from build123d import *

# Parameters (mm, degrees)
SKETCH1_W                 = 40
SKETCH1_H                 = 20
BOSS_EXTRUDE1_DEPTH       = 38
BOSS_EXTRUDE2_DEPTH       = 2
BOSS_EXTRUDE3_DEPTH       = 0.5
SKETCH6_W                 = 12.8
SKETCH6_H                 = 17.8
SKETCH6_W_2               = 10.8
SKETCH6_H_2               = 15.8
BOSS_EXTRUDE4_DEPTH       = 0.5
BOSS_EXTRUDE5_DEPTH       = 0.5
SKETCH8_R                 = 6.5
BOSS_EXTRUDE6_DEPTH       = 1
SKETCH9_R                 = 5.25
BOSS_EXTRUDE7_DEPTH       = 0.5
SKETCH10_R                = 3
BOSS_EXTRUDE8_DEPTH       = 4
SKETCH11_R                = 1.5
CUT_EXTRUDE1_DEPTH        = 10
CHAMFER1_SIZE             = 2
SKETCH12_R                = 2
CUT_EXTRUDE2_DEPTH        = 2
FILLET1_R                 = 0.5
FILLET2_R                 = 0.25
BOSS_EXTRUDE9_DEPTH       = 2.4
BOSS_EXTRUDE10_DEPTH      = 0.5
BOSS_EXTRUDE10_DEPTH_BACK = 0.5
FILLET3_R                 = 1.5


with BuildPart() as part:
    # Sketch1 → Boss-Extrude1 (new body)
    with BuildSketch(Plane(origin=(0, 0, 0), x_dir=(1, 0, 0), z_dir=(0, 1, 0))):
        Rectangle(SKETCH1_W, SKETCH1_H)
    extrude(amount=BOSS_EXTRUDE1_DEPTH)

    # Sketch2 → Boss-Extrude2 (add)
    with BuildSketch(Plane(origin=(0, 38, 0), x_dir=(1, 0, 0), z_dir=(0, 1, 0))):
        with BuildLine():
            ThreePointArc((-3.783333333, 0), (-7.418581742, 5.77726026), (-14.2, 5))
            Line((-14.2, 5), (-14.2, -5))
            ThreePointArc((-14.2, -5), (-7.418581742, -5.77726026), (-3.783333333, 0))
        make_face()
        with BuildLine():
            Line((-14.2, -5), (-14.2, 5))
            ThreePointArc((-14.2, 5), (-16.6, 0), (-14.2, -5))
        make_face()
        with BuildLine():
            Line((5.440394754, 8.9), (-14.2, 8.9))
            Line((-14.2, 8.9), (-14.2, 5))
            ThreePointArc((-14.2, 5), (-7.418581742, 5.77726026), (-3.783333333, 0))
            ThreePointArc((-3.783333333, 0), (-7.418581742, -5.77726026), (-14.2, -5))
            Line((-14.2, -5), (-14.2, -8.9))
            Line((-14.2, -8.9), (5.440394754, -8.9))
            ThreePointArc((5.440394754, -8.9), (0, 0), (5.440394754, 8.9))
        make_face()
        with BuildLine():
            ThreePointArc((20, 0), (15.215551147, 8.532175938), (5.440394754, 8.9))
            Line((5.440394754, 8.9), (5.440394754, -8.9))
            ThreePointArc((5.440394754, -8.9), (15.215551147, -8.532175938), (20, 0))
        make_face()
        with BuildLine():
            Line((5.440394754, -8.9), (5.440394754, 8.9))
            ThreePointArc((5.440394754, 8.9), (0, 0), (5.440394754, -8.9))
        make_face()
    extrude(amount=BOSS_EXTRUDE2_DEPTH)

    # Sketch3 → Boss-Extrude3 (add)
    with BuildSketch(Plane(origin=(0, 38, 0), x_dir=(1, 0, 0), z_dir=(0, 1, 0))):
        Polygon((-19.65, 9.65), (10, 9.65), (19.65, 9.65), (19.65, 0), (19.65, -9.65), (10, -9.65), (-19.65, -9.65), align=None)
    extrude(amount=BOSS_EXTRUDE3_DEPTH)

    # Sketch6 → Boss-Extrude4 (add)
    with BuildSketch(Plane(origin=(0, 40, 0), x_dir=(1, 0, 0), z_dir=(0, 1, 0))):
        with Locations((-7.8, 0)):
            Rectangle(SKETCH6_W, SKETCH6_H)
        with Locations((-7.8, 0)):
            Rectangle(SKETCH6_W_2, SKETCH6_H_2, mode=Mode.SUBTRACT)
    extrude(amount=BOSS_EXTRUDE4_DEPTH)

    # Sketch7 → Boss-Extrude5 (add)
    with BuildSketch(Plane(origin=(0, 40, 0), x_dir=(1, 0, 0), z_dir=(0, 1, 0))):
        with BuildLine():
            ThreePointArc((0.6, 0), (0.014213562, 1.414213562), (-1.4, 2))
            Line((-1.4, 2), (-1.4, -2))
            ThreePointArc((-1.4, -2), (0.014213562, -1.414213562), (0.6, 0))
        make_face()
    extrude(amount=BOSS_EXTRUDE5_DEPTH)

    # Sketch8 → Boss-Extrude6 (add)
    with BuildSketch(Plane(origin=(0, 40, 0), x_dir=(1, 0, 0), z_dir=(0, 1, 0))):
        with Locations(Location((10, 0, 0), (0, 0, 270))):
            Circle(SKETCH8_R)
    extrude(amount=BOSS_EXTRUDE6_DEPTH)

    # Sketch9 → Boss-Extrude7 (add)
    with BuildSketch(Plane(origin=(0, 41, 0), x_dir=(1, 0, 0), z_dir=(0, 1, 0))):
        with Locations(Location((10, 0, 0), (0, 0, 270))):
            Circle(SKETCH9_R)
    extrude(amount=BOSS_EXTRUDE7_DEPTH)

    # Sketch10 → Boss-Extrude8 (add)
    with BuildSketch(Plane(origin=(0, 41.5, 0), x_dir=(1, 0, 0), z_dir=(0, 1, 0))):
        with Locations(Location((10, 0, 0), (0, 0, 270))):
            Circle(SKETCH10_R)
    extrude(amount=BOSS_EXTRUDE8_DEPTH)

    # Sketch11 → Cut-Extrude1 (cut)
    with BuildSketch(Plane(origin=(0, 45.5, 0), x_dir=(1, 0, 0), z_dir=(0, 1, 0))):
        with Locations(Location((10, 0, 0), (0, 0, 270))):
            Circle(SKETCH11_R)
    extrude(amount=-CUT_EXTRUDE1_DEPTH, mode=Mode.SUBTRACT)

    # Chamfer1
    chamfer1_edges = [part.edges().sort_by_distance(p)[0] for p in [
        (-20, 0, 0),
        (0, 0, 10),
        (20, 0, 0),
        (0, 0, -10),
    ]]
    chamfer(chamfer1_edges, length=CHAMFER1_SIZE)

    # Sketch12 → Cut-Extrude2 (cut)
    with BuildSketch(Plane.XZ):
        with Locations((19, 9)):
            Circle(SKETCH12_R)
        with Locations((-19, 9)):
            Circle(SKETCH12_R)
        with Locations((19, -9)):
            Circle(SKETCH12_R)
        with Locations((-19, -9)):
            Circle(SKETCH12_R)
    extrude(amount=-CUT_EXTRUDE2_DEPTH, mode=Mode.SUBTRACT)

    # Fillet1
    fillet1_edges = [part.edges().sort_by_distance(p)[0] for p in [
        (-20, 20, -10),
        (-20, 20, 10),
        (20, 20, 10),
        (20, 20, -10),
    ]]
    fillet(fillet1_edges, radius=FILLET1_R)

    # Fillet2
    fillet2_edges = [part.edges().sort_by_distance(p)[0] for p in [
        (5.440394754, 39.25, 8.9),
        (5.440394754, 39.25, -8.9),
        (7.377501192, 38.25, 9.65),
        (7.377501192, 38.25, -9.65),
        (12.622498808, 38.25, -9.65),
        (19.65, 38.25, -2.622498808),
        (19.65, 38.25, 2.622498808),
        (12.622498808, 38.25, 9.65),
        (-19.65, 38.25, 9.65),
        (19.65, 38.25, 9.65),
        (19.65, 38.25, -9.65),
        (-19.65, 38.25, -9.65),
    ]]
    fillet(fillet2_edges, radius=FILLET2_R)

    # Sketch13 → Boss-Extrude9 (add)
    with BuildSketch(Plane(origin=(0, 32.8, 0), x_dir=(1, 0, 0), z_dir=(0, 1, 0))):
        with BuildLine():
            Line((-20, -9.5), (-20, 9.5))
            Line((-20, 9.5), (-26.8, 9.5))
            Line((-26.8, 9.5), (-26.8, 6.2))
            Line((-26.8, 6.2), (-26.243908891, 6.2))
            ThreePointArc((-26.243908891, 6.2), (-23.774140416, 7.109099282), (-22.2, 5))
            ThreePointArc((-22.2, 5), (-23.774140416, 2.890900718), (-26.243908891, 3.8))
            Line((-26.243908891, 3.8), (-26.8, 3.8))
            Line((-26.8, 3.8), (-26.8, -3.8))
            Line((-26.8, -3.8), (-26.243908891, -3.8))
            ThreePointArc((-26.243908891, -3.8), (-23.774140416, -2.890900718), (-22.2, -5))
            ThreePointArc((-22.2, -5), (-23.774140416, -7.109099282), (-26.243908891, -6.2))
            Line((-26.243908891, -6.2), (-26.8, -6.2))
            Line((-26.8, -6.2), (-26.8, -9.5))
            Line((-26.8, -9.5), (-20, -9.5))
        make_face()
        with BuildLine():
            Line((26.243908891, 6.2), (26.8, 6.2))
            Line((26.8, 6.2), (26.8, 9.5))
            Line((26.8, 9.5), (20, 9.5))
            Line((20, 9.5), (20, -9.5))
            Line((20, -9.5), (26.8, -9.5))
            Line((26.8, -9.5), (26.8, -6.2))
            Line((26.8, -6.2), (26.243908891, -6.2))
            ThreePointArc((26.243908891, -6.2), (22.2, -5), (26.243908891, -3.8))
            Line((26.243908891, -3.8), (26.8, -3.8))
            Line((26.8, -3.8), (26.8, 3.8))
            Line((26.8, 3.8), (26.243908891, 3.8))
            ThreePointArc((26.243908891, 3.8), (22.2, 5), (26.243908891, 6.2))
        make_face()
    extrude(amount=-BOSS_EXTRUDE9_DEPTH)

    # Sketch14 → Boss-Extrude10 (add, two sides: drawn at the far end of the back side and taken through both)
    with BuildSketch(Plane.XY.offset(-BOSS_EXTRUDE10_DEPTH_BACK)):
        Polygon((-26.8, 32.8), (-20, 32.8), (-20, 34.3), align=None)
        Polygon((20, 32.8), (20, 34.3), (26.8, 32.8), align=None)
    extrude(amount=BOSS_EXTRUDE10_DEPTH + BOSS_EXTRUDE10_DEPTH_BACK)

    # Fillet3
    fillet3_edges = [part.edges().sort_by_distance(p)[0] for p in [
        (-26.8, 31.6, -9.5),
        (-26.8, 31.6, 9.5),
        (26.8, 31.6, 9.5),
        (26.8, 31.6, -9.5),
    ]]
    fillet(fillet3_edges, radius=FILLET3_R)


solid = part.part
Source: CAD feature listing. Evaluate the final solid. Frame: model axes, mm. A direction names the side the tool comes from. Round coordinates to 2 decimals unless told otherwise and drop trailing zeros. Loops run counter-clockwise (first coordinate to the right, second up) from the corner with the lowest first, then second, coordinate; pieces in that order, holes last. Notation, with made-up numbers: (71, -28.75) - (84, -28.75) arc R6 ccw to (84, -22.75) - close; hole circle Ø2 at (80.5, -10). An arc over 180 degrees is marked (long way). Write item = value, one per line. Start each with the question number.
(1) Section query A-A, the plane x = -10.5. Output: boundary loops of the cut face in (y, z), plus the area to 3 significant figures.
(2) Section query C-C, the plane y = 33.5. Output: boundary loops of the cut face in (x, z), plus the area to 3 significant figures.
(3) Ray query, line 1 along Z through (x, y) = (24.4, 31.65); line 2 along X through (y, z) = (41.25, 0); line 3 along X through (y, z) = (42.5, 0). Return the intervals inside material, ascending. Write a range as from..to.
(4) Pin query (flat end, axial travel): pin 1 (1.8 mm diameter, centred on x = 10, z = 0, fed in from +Y); pin 2 (0.9 mm diameter, centred on x = 18.5, z = -9, fed in from -Y); pin 3 (2.5 mm diameter, centred on x = -23, y = 32, fed in from -Z). Return the tip coordinate at first contact, or that it passes through.
(5) Pull-direction query (X, two-part tool) for faces 1 (the face through (20, 16, 0)), 2 (the face through (0, 0, 0)), 3 (the face through (22.2, 31.62, -4.92)); classes: +X half, -X half, draft (parallel to the pull), parting line (faces both ways), or undercut.
(6) Section query B-B, the plane x = 24.4. Output: boundary loops of the cut face in (y, z), plus the area to 3 significant figures.
(7) Set-up query: faces 4 (the face through (22, 33, 0.5)), 5 (the face through (17.61, 1.21, -7.56)), 6 (the face through (-22, 32.8, -5)). Return all of +Z, -Z, +X, -X, +Y, -Y with unobstructed straight access to the full face (end or side cutting, diameter ignored); none if empty.
Conclusion:
q1.outline = (0, -8) - (2, -10) - (38, -10) - (38, -9.65) - (38.5, -9.65) - (38.5, -8.9) - (40.5, -8.9) - (40.5, -7.9) - (40, -7.9) - (40, 7.9) - (40.5, 7.9) - (40.5, 8.9) - (38.5, 8.9) - (38.5, 9.65) - (38, 9.65) - (38, 10) - (2, 10) - (0, 8) - close
q1.area = 793 mm2
q2.outline = (-23.63, -0.5) - (-20, -0.5) - (-20, -9.5) arc R0.5 ccw to (-19.5, -10) - (19.5, -10) arc R0.5 ccw to (20, -9.5) - (20, -0.5) - (23.63, -0.5) - (23.63, 0.5) - (20, 0.5) - (20, 9.5) arc R0.5 ccw to (19.5, 10) - (-19.5, 10) arc R0.5 ccw to (-20, 9.5) - (-20, 0.5) - (-23.63, 0.5) - close
q2.area = 807 mm2
q3.line_1 = -9.5..-7.2, -2.8..2.8, 7.2..9.5
q3.line_2 = 4.75..8.5, 11.5..15.25
q3.line_3 = 7..8.5, 11.5..13
q4.pin_1 = 35.5
q4.pin_2 = 2
q4.pin_3 = -9.5
q5.face_1 = +X half
q5.face_2 = draft
q5.face_3 = undercut
q6.outline = (30.4, -9.5) - (32.8, -9.5) - (32.8, -7.2) - (30.4, -7.2) - close; (30.4, -2.8) - (32.8, -2.8) - (32.8, -0.5) - (33.33, -0.5) - (33.33, 0.5) - (32.8, 0.5) - (32.8, 2.8) - (30.4, 2.8) - close; (30.4, 7.2) - (32.8, 7.2) - (32.8, 9.5) - (30.4, 9.5) - close
q6.area = 25.0 mm2
q7.face_4 = +Z, +X, +Y
q7.face_5 = -Y
q7.face_6 = -Z, -X, +Y
